CAD build for the part. Positions are in the model's coordinates, mm. Face numbers are marked on the shaded views. A direction names the side the tool comes from. Coordinates: 2 decimals unless noted, no trailing zeros. Write each loop counter-clockwise with the first axis right and the second up, starting at its lowest first coordinate (ties: lowest second). Pieces come first, ordered by that corner, then holes. Notation, with made-up numbers: (85.25, -10.75) - (124.25, -10.75) arc R28 ccw to (124.25, 16.25) - close; hole circle Ø8 at (-7.5, -11.75). An arc over 180 degrees is marked (long way). One line per question, with ' | ' between items. Start each with the question number.
1. Band-saw the part on C-C, the plane z = 17.5. Write the cut outline in (x, y).
2. Flat gauge pins, fed straight in: P1, Ø1.6, axis at y = 15, z = -3, coming from the -X side; P2, Ø1.2, axis at y = 17, z = 20, coming from the +X side; P3, Ø1.6, axis at y = 14.5, z = 17.5, coming from the -X side. Where does each tip first touch, or does it go through?
3. Band-saw the part on B-B, the plane x = -20. Write the cut outline in (y, z), then the cut area to 3 significant figures.
4. Two-plate mould, pull along Z, no slides. Class the marked faces 3, 4 and 5: +Z half, -Z half, draft (parallel to the pull), parting line (faces both ways), or undercut.
5. Probe line 1 (Z direction, x = -29.5, y = 16); line 2 (Y direction, x = -28, z = -19); line 3 (X direction, y = 7.5, z = 1). List the from-to ranges inside material, lowest first.
6. Band-saw the part on A-A, the plane z = 5. Write the cut outline in (x, y), then the cut area to 3 significant figures.
7. Which spindle directions (+Z, -Z, +X, -X, +Y, -Y) get a long thin tool onto all of the face, cutting with end or side? Do the marked faces 1 and 2. Say none if no direction does.
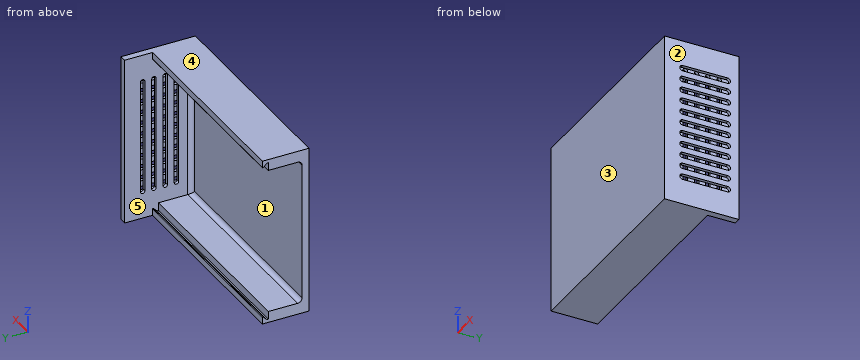
from build123d import *

# Parameters (mm, degrees)
SKETCH1_W           = 95
SKETCH1_H           = 75
BOSS_EXTRUDE1_DEPTH = 3
SKETCH2_W           = 95
SKETCH2_H           = 5
BOSS_EXTRUDE2_DEPTH = 15
SKETCH3_W           = 3
SKETCH3_H           = 75
BOSS_EXTRUDE3_DEPTH = 30
CUT_EXTRUDE1_DEPTH  = 1.5
CUT_EXTRUDE2_DEPTH  = 1.5
BOSS_EXTRUDE4_DEPTH = 95
FILLET1_R           = 0.2
FILLET2_R           = 2


with BuildPart() as part:
    # Sketch1 → Boss-Extrude1 (new body)
    with BuildSketch(Plane(origin=(0, 0, 0), x_dir=(1, 0, 0), z_dir=(0, 1, 0))):
        Rectangle(SKETCH1_W, SKETCH1_H)
    extrude(amount=BOSS_EXTRUDE1_DEPTH)

    # Sketch2 → Boss-Extrude2 (add)
    with BuildSketch(Plane(origin=(0, 3, 0), x_dir=(1, 0, 0), z_dir=(0, 1, 0))):
        with Locations((0, 35)):
            Rectangle(SKETCH2_W, SKETCH2_H)
        with Locations((0, -35)):
            Rectangle(SKETCH2_W, SKETCH2_H)
    extrude(amount=BOSS_EXTRUDE2_DEPTH)

    # Sketch3 → Boss-Extrude3 (add)
    with BuildSketch(Plane(origin=(0, 3, 0), x_dir=(1, 0, 0), z_dir=(0, 1, 0))):
        with Locations((46, 0)):
            Rectangle(SKETCH3_W, SKETCH3_H)
    extrude(amount=BOSS_EXTRUDE3_DEPTH)

    # Sketch4 → Cut-Extrude1 (cut)
    with BuildSketch(Plane(origin=(47.5, 0, 0), x_dir=(0, 0, -1), z_dir=(1, 0, 0))):
        with BuildLine():
            Line((26.25, 8), (26.25, 28))
            ThreePointArc((26.25, 28), (25, 29.25), (23.75, 28))
            Line((23.75, 28), (23.75, 8))
            ThreePointArc((23.75, 8), (25, 6.75), (26.25, 8))
        make_face()
        with BuildLine():
            Line((21.25, 8), (21.25, 28))
            ThreePointArc((21.25, 28), (20, 29.25), (18.75, 28))
            Line((18.75, 28), (18.75, 8))
            ThreePointArc((18.75, 8), (20, 6.75), (21.25, 8))
        make_face()
        with BuildLine():
            Line((16.25, 8), (16.25, 28))
            ThreePointArc((16.25, 28), (15, 29.25), (13.75, 28))
            Line((13.75, 28), (13.75, 8))
            ThreePointArc((13.75, 8), (15, 6.75), (16.25, 8))
        make_face()
        with BuildLine():
            Line((11.25, 8), (11.25, 28))
            ThreePointArc((11.25, 28), (10, 29.25), (8.75, 28))
            Line((8.75, 28), (8.75, 8))
            ThreePointArc((8.75, 8), (10, 6.75), (11.25, 8))
        make_face()
        with BuildLine():
            Line((6.25, 8), (6.25, 28))
            ThreePointArc((6.25, 28), (5, 29.25), (3.75, 28))
            Line((3.75, 28), (3.75, 8))
            ThreePointArc((3.75, 8), (5, 6.75), (6.25, 8))
        make_face()
        with BuildLine():
            Line((1.25, 8), (1.25, 28))
            ThreePointArc((1.25, 28), (0, 29.25), (-1.25, 28))
            Line((-1.25, 28), (-1.25, 8))
            ThreePointArc((-1.25, 8), (0, 6.75), (1.25, 8))
        make_face()
        with BuildLine():
            Line((-3.75, 8), (-3.75, 28))
            ThreePointArc((-3.75, 28), (-5, 29.25), (-6.25, 28))
            Line((-6.25, 28), (-6.25, 8))
            ThreePointArc((-6.25, 8), (-5, 6.75), (-3.75, 8))
        make_face()
        with BuildLine():
            Line((-8.75, 8), (-8.75, 28))
            ThreePointArc((-8.75, 28), (-10, 29.25), (-11.25, 28))
            Line((-11.25, 28), (-11.25, 8))
            ThreePointArc((-11.25, 8), (-10, 6.75), (-8.75, 8))
        make_face()
        with BuildLine():
            Line((-13.75, 8), (-13.75, 28))
            ThreePointArc((-13.75, 28), (-15, 29.25), (-16.25, 28))
            Line((-16.25, 28), (-16.25, 8))
            ThreePointArc((-16.25, 8), (-15, 6.75), (-13.75, 8))
        make_face()
        with BuildLine():
            Line((-18.75, 8), (-18.75, 28))
            ThreePointArc((-18.75, 28), (-20, 29.25), (-21.25, 28))
            Line((-21.25, 28), (-21.25, 8))
            ThreePointArc((-21.25, 8), (-20, 6.75), (-18.75, 8))
        make_face()
        with BuildLine():
            Line((-23.75, 8), (-23.75, 28))
            ThreePointArc((-23.75, 28), (-25, 29.25), (-26.25, 28))
            Line((-26.25, 28), (-26.25, 8))
            ThreePointArc((-26.25, 8), (-25, 6.75), (-23.75, 8))
        make_face()
    extrude(amount=-CUT_EXTRUDE1_DEPTH, mode=Mode.SUBTRACT)

    # Sketch5 → Cut-Extrude2 (cut)
    with BuildSketch(Plane.ZY.offset(-44.5)):
        with BuildLine():
            Line((-25.25, 24), (25.25, 24))
            ThreePointArc((25.25, 24), (26.25, 25), (25.25, 26))
            Line((25.25, 26), (-25.25, 26))
            ThreePointArc((-25.25, 26), (-26.25, 25), (-25.25, 24))
        make_face()
        with BuildLine():
            Line((-25.25, 19), (25.25, 19))
            ThreePointArc((25.25, 19), (26.25, 20), (25.25, 21))
            Line((25.25, 21), (-25.25, 21))
            ThreePointArc((-25.25, 21), (-26.25, 20), (-25.25, 19))
        make_face()
        with BuildLine():
            Line((-25.25, 14), (25.25, 14))
            ThreePointArc((25.25, 14), (26.25, 15), (25.25, 16))
            Line((25.25, 16), (-25.25, 16))
            ThreePointArc((-25.25, 16), (-26.25, 15), (-25.25, 14))
        make_face()
        with BuildLine():
            Line((-25.25, 9), (25.25, 9))
            ThreePointArc((25.25, 9), (26.25, 10), (25.25, 11))
            Line((25.25, 11), (-25.25, 11))
            ThreePointArc((-25.25, 11), (-26.25, 10), (-25.25, 9))
        make_face()
    extrude(amount=-CUT_EXTRUDE2_DEPTH, mode=Mode.SUBTRACT)

    # Sketch6 → Boss-Extrude4 (add)
    with BuildSketch(Plane.ZY.offset(47.5)):
        Polygon((37.5, 18), (37.5, 20.65), (34.05, 20.65), (36.05, 18.65), (36.05, 18), align=None)
        Polygon((-36.05, 18), (-37.5, 18), (-37.5, 20.65), (-34.05, 20.65), (-36.05, 18.65), align=None)
    extrude(amount=-BOSS_EXTRUDE4_DEPTH)

    # Fillet1
    fillet1_edges = [part.edges().sort_by_distance(p)[0] for p in [
        (-1.5, 20.65, 34.05),
        (-1.5, 20.65, -34.05),
    ]]
    fillet(fillet1_edges, radius=FILLET1_R)

    # Fillet2
    fillet2_edges = [part.edges().sort_by_distance(p)[0] for p in [
        (-1.5, 3, -32.5),
        (-1.5, 3, 32.5),
        (44.5, 3, 0),
    ]]
    fillet(fillet2_edges, radius=FILLET2_R)


solid = part.part
Filled in:
1) outline: (-47.5, 0) - (47.5, 0) - (47.5, 33) - (44.5, 33) - (44.5, 26) - (46, 26) - (46, 24) - (44.5, 24) - (44.5, 21) - (46, 21) - (46, 19) - (44.5, 19) - (44.5, 16) - (46, 16) - (46, 14) - (44.5, 14) - (44.5, 11) - (46, 11) - (46, 9) - (44.5, 9) - (44.5, 5) arc R2 cw to (42.5, 3) - (-47.5, 3) - close
2) P1: stops at x = 46 | P2: stops at x = 46 | P3: stops at x = 44.5
3) outline: (0, -37.5) - (20.65, -37.5) - (20.65, -34.53) arc R0.2 ccw to (20.31, -34.39) - (18.65, -36.05) - (18, -36.05) - (18, -32.5) - (5, -32.5) arc R2 cw to (3, -30.5) - (3, 30.5) arc R2 cw to (5, 32.5) - (18, 32.5) - (18, 36.05) - (18.65, 36.05) - (20.31, 34.39) arc R0.2 ccw to (20.65, 34.53) - (20.65, 37.5) - (0, 37.5) - close | area: 388 mm²
4) face 3: draft | face 4: +Z half | face 5: undercut
5) line 1: z = -37.5 to -32.5, 32.5 to 37.5 | line 2: y = 0 to 3 | line 3: x = 44.5 to 46
6) outline: (-47.5, 0) - (47.5, 0) - (47.5, 6.75) - (46, 6.75) - (46, 9) - (44.5, 9) - (44.5, 5) arc R2 cw to (42.5, 3) - (-47.5, 3) - close; (44.5, 11) - (46, 11) - (46, 14) - (44.5, 14) - close; (44.5, 16) - (46, 16) - (46, 19) - (44.5, 19) - close; (44.5, 21) - (46, 21) - (46, 24) - (44.5, 24) - close; (44.5, 26) - (46, 26) - (46, 29.25) - (47.5, 29.25) - (47.5, 33) - (44.5, 33) - close | area: 330 mm²
7) face 1: -X, +Y | face 2: +Z, -Z, +X, +Y, -Y
